from build123d import *

# Parameters (mm, degrees)
BOSS_EXTRUDE1_DEPTH = 3.429
FILLET1_R           = 3.175
SHELL1_START        = 0.762
SHELL1_DEPTH        = 2.667
SKETCH2_R           = 2.1717
SKETCH2_R_2         = 3.3274
CUT_EXTRUDE1_DEPTH  = 109.116950745
SKETCH4_W           = 1.905
SKETCH4_H           = 37.1856
CUT_EXTRUDE3_DEPTH  = 8.509


# Read off the part's stored shape, not the designer's step: Shell1
with BuildPart() as part:
    # Sketch1 → Boss-Extrude1 (new body)
    with BuildSketch(Plane.XY):
        with BuildLine():
            Line((62.694975666, 80.659735828), (64.726975666, 62.193935828))
            ThreePointArc((64.726975666, 62.193935828), (62.449213934, 49.504733029), (61.678975666, 36.635747087))
            ThreePointArc((61.678975666, 36.635747087), (63.002494237, 30.6317877), (66.736169072, 25.747230203))
            Line((66.736169072, 25.747230203), (68.652274874, 13.809230203))
            Line((68.652274874, 13.809230203), (56.968274874, 15.553747087))
            ThreePointArc((56.968274874, 15.553747087), (52.42740055, 32.785925059), (52.280975666, 50.605747087))
            Line((52.280975666, 50.605747087), (53.296975666, 64.575747087))
            ThreePointArc((53.296975666, 64.575747087), (53.599423451, 70.100985632), (52.031009659, 75.407567754))
            ThreePointArc((52.031009659, 75.407567754), (54.734890855, 83.369731663), (62.694975666, 80.659735828))
        make_face()
    extrude(amount=BOSS_EXTRUDE1_DEPTH)

    # Fillet1
    fillet1_edges = [part.edges().sort_by_distance(p)[0] for p in [
        (68.652274874, 13.809230203, 1.7145),
    ]]
    fillet(fillet1_edges, radius=FILLET1_R)

    # Shell1 outline → Shell1 (cut)
    with BuildSketch(Plane.XY.offset(SHELL1_START)):
        with BuildLine():
            ThreePointArc((61.952685119, 80.438826605), (55.013786801, 82.65723656), (52.714338634, 75.744770233))
            ThreePointArc((52.714338634, 75.744770233), (54.352815027, 70.218797874), (54.052777411, 64.462848531))
            Line((54.052777411, 64.462848531), (53.039751684, 50.533744782))
            ThreePointArc((53.039751684, 50.533744782), (53.153060273, 33.111126197), (57.513949579, 16.242720176))
            Line((57.513949579, 16.242720176), (64.473451012, 15.203609619))
            ThreePointArc((64.473451012, 15.203609619), (66.545332993, 15.893259626), (67.212288081, 17.972558303))
            Line((67.212288081, 17.972558303), (66.027992544, 25.351127953))
            ThreePointArc((66.027992544, 25.351127953), (62.25173003, 30.440896905), (60.916975951, 36.636406417))
            ThreePointArc((60.916975951, 36.636406417), (61.6846952, 49.528718986), (63.955003411, 62.242759133))
            Line((63.955003411, 62.242759133), (61.952685119, 80.438826605))
        make_face()
    extrude(amount=SHELL1_DEPTH, mode=Mode.SUBTRACT)

    # Sketch2 → Cut-Extrude1 (cut, through all)
    with BuildSketch(Plane.XY.offset(3.429)):
        with Locations((57.360975666, 78.037747087)):
            Circle(SKETCH2_R)
        with Locations((63.072884184, 19.881317109)):
            Circle(SKETCH2_R_2)
    extrude(amount=-CUT_EXTRUDE1_DEPTH, mode=Mode.SUBTRACT)

    # Sketch4 → Cut-Extrude3 (cut)
    with BuildSketch(Plane(origin=(70.714586477, 7.781522583, 0), x_dir=(0, 0, -1), z_dir=(0.9939998970848155, 0.1093810065567881, 0))):
        with Locations((-2.4765, 36.148064063)):
            Rectangle(SKETCH4_W, SKETCH4_H)
    extrude(amount=-CUT_EXTRUDE3_DEPTH, mode=Mode.SUBTRACT)


solid = part.part
Check sheet for the modelled part. Datum: model origin and axes. Units: mm. A direction names the side the tool comes from. Give positions to 0.01 mm unless a question says otherwise; leave off trailing zeros. Loops run counter-clockwise (first coordinate to the right, second up) from the corner with the lowest first, then second, coordinate; pieces in that order, holes last. Notation, with made-up numbers: M 21.25,66 L 71.25,66 A26 ccw 71.25,96 Z; hole C -10.5,-5 d7. An arc over 180 degrees is marked long. Answer as a JSON object with one key per item and string values. Group by question number.
Q1. Go/stop test with flat-tipped pins: P1, Ø3, axis at x = 63, y = 46, coming from the +Z side; P2, Ø4.5, axis at x = 58, y = 42.5, coming from the +Z side; P3, Ø1.5, axis at x = 60.5, z = 0.5, coming from the -Y side. Record where each tip stops, or that it passes through.
Q2. Cross-section at B-B on y = 19. Record the cut outline in (x, z), then the cut area to 3 significant figures.
Q3. Release check for a two-part mould opening along Y. For faces 6 (the cylindrical face through (55.1, 82.7, 2.1)), 7 (the flat face through (67.342, 21.974, 1.69)), 8 (the flat face through (58, 50, 0)) record: released by +Y, released by -Y, zero draft, split by the parting line, or undercut.
Q4. Cross-section at D-D on y = 28.5. Record the cut outline in (x, z).
Q5. Access from +Z, -Z, +X, -X, +Y, -Y to the whole of each face (thin tool, end or side, straight path). Record for faces 1 (the flat face through (52.78, 57.49, 1.69)), 2 (the cylindrical face through (66.247, 20.881, 0.386)), 3 (the cylindrical face through (62.29, 30.36, 1.14)), 4 (the flat face through (63.697, 71.556, 1.69)), 5 (the cylindrical face through (62.47, 49.68, 0.75)).
Q6. Cross-section at C-C on y = 40. Record the cut outline in (x, z).
Q7. Material ranges on line 1 along Z through (x, y) = (65.5, 25.5); line 2 along Y through (x, z) = (59.75, 0.85); line 3 along X through (y, z) = (65, 1.9), recorded low to high. Write a range as [from, to].
Evaluation:
{
 "1": {"P1": "stops at z = 1.52", "P2": "stops at z = 0.76", "P3": "stops at y = 14.91"},
 "2": {"outline": "M 55.68,0 L 59.86,0 L 59.86,0.76 L 56.49,0.76 L 56.49,3.43 L 55.68,3.43 Z; M 66.28,0 L 67.82,0 L 67.82,3.43 L 67.05,3.43 L 67.05,0.76 L 66.28,0.76 Z", "area": "8.57 mm2"},
 "3": {"face 6": "undercut", "face 7": "released by +Y", "face 8": "zero draft"},
 "4": {"outline": "M 53.13,0 L 64.23,0 L 64.23,1.52 L 63.31,1.52 L 63.31,0.76 L 53.91,0.76 L 53.91,3.43 L 53.13,3.43 Z"},
 "5": {"face 1": "+Z, -Z, -X", "face 2": "+Z, -Z", "face 3": "+Z", "face 4": "+Z, -Z, +X, +Y", "face 5": "+Z, -Z, +X"},
 "6": {"outline": "M 51.83,0 L 61.73,0 L 61.73,1.52 L 60.97,1.52 L 60.97,0.76 L 52.59,0.76 L 52.59,3.43 L 51.83,3.43 Z"},
 "7": {"line 1": "z = [0, 0.76]", "line 2": "y = [15.14, 15.91], [82.64, 83.48]", "line 3": "x = [53.39, 54.17], [63.65, 64.42]"}
}
